from build123d import *

# Parameters (mm, degrees)
F3_DEPTH = 1.5
F4_R     = 4
F5_DEPTH = 0.5


with BuildPart() as f3:
    # F2 (on Top) → F3 (new body)
    with BuildSketch(Plane.XY):
        with BuildLine():
            ThreePointArc((0.3102344361, 4.9903661784), (-3.6435677694, -3.4240931515), (5, 0))
            ThreePointArc((5, 0), (4.8674688244, 1.1435677694), (4.4769011027, 2.2265121865))
            Line((4.4769011027, 2.2265121865), (1.5, 0))
            ThreePointArc((1.5, 0), (-0.8291561976, -1.25), (-0.5833333333, 1.381926996))
            Line((-0.5833333333, 1.381926996), (0.3102344361, 4.9903661784))
        make_face()
    extrude(amount=F3_DEPTH)

    # F4 (on face) → F5 (cut)
    with BuildSketch(Plane.XY.offset(1.5)):
        Circle(F4_R)
    extrude(amount=F5_DEPTH, mode=Mode.SUBTRACT)


solid = f3.part
The model under review builds one solid part; all positions refer to its coordinate system, in mm. A direction names the side the tool comes from. Coordinates: 2 decimals unless noted, no trailing zeros. Loops run counter-clockwise (first coordinate to the right, second up) from the corner with the lowest first, then second, coordinate; pieces in that order, holes last.
(1) Wall thickness on L1, parallel to Y at x = -1, z = 0.55; L2, parallel to X at y = 3, z = 1.4; L3, parallel to X at y = -0.25, z = 1.4: over which ranges is each line inside the solid? List them lowest first.
Determined:
L1: y = -4.9 to -1.12, 1.12 to 4.9
L2: x = -4 to -0.18
L3: x = -4.99 to -1.48, 1.48 to 4.99
(2) Consider section C-C, the plane z = 0.3. Give the boundary of the cut face in (x, y), plus the area to 3 significant figures.
Determined:
outline: (-0.58, 1.38) - (0.31, 4.99) arc R5 ccw (long way) to (4.48, 2.23) - (1.5, 0) arc R1.5 cw (long way) to start
area: 57.3 mm2
(3) Consider section B-B, the plane y = 0.25. Give the boundary of the cut face in (x, z), plus the area to 3 significant figures.
Determined:
outline: (-4.99, 0) - (-1.48, 0) - (-1.48, 1.5) - (-4.99, 1.5) - close; (1.83, 0) - (4.99, 0) - (4.99, 1.5) - (1.83, 1.5) - close
area: 10.0 mm2
(4) Tool access review of faces 1 (the flat face through (0, -2, 1.5)), 2 (the flat face through (-0.143, 3.161, 0.74)): name each direction out of +Z, -Z, +X, -X, +Y, -Y from which nothing blocks a thin tool from reaching the whole face with its end or side.
Determined:
face 1: +Z, +X, -X, +Y, -Y
face 2: +Z, -Z
(5) Consider section A-A, the plane x = 0. Give the boundary of the cut face in (y, z).
Determined:
outline: (-5, 0) - (-1.5, 0) - (-1.5, 1.5) - (-5, 1.5) - close; (3.74, 0) - (5, 0) - (5, 1.5) - (3.74, 1.5) - close
(6) Consider section D-D, the plane x = 2. Give the boundary of the cut face in (y, z).
Determined:
outline: (-4.58, 0) - (0.37, 0) - (0.37, 1.5) - (-4.58, 1.5) - close
(7) Draft analysis for pull direction X (two halves, no side actions). For faces 3 (the flat face through (3.01, 1.13, 0.74)), 4 (the flat face through (0, -2, 0)), state which applies: +X half, -X half, draft (parallel to the pull), parting line (faces both ways), or undercut.
Determined:
face 3: undercut
face 4: draft
